```python
from build123d import *

# Parameters (mm, degrees)
BOSS_EXTRUDE1_DEPTH = 17
SKETCH3_R           = 3.25
CUT_EXTRUDE1_DEPTH  = 6
SKETCH4_R           = 3
BOSS_EXTRUDE2_DEPTH = 8


with BuildPart() as part:
    # Sketch2 → Boss-Extrude1 (new body)
    with BuildSketch(Plane.XY):
        with BuildLine():
            Line((-50.590688259, -20.348178138), (79.409311741, -20.348178138))
            ThreePointArc((79.409311741, -20.348178138), (86.480379553, -17.41924595), (89.409311741, -10.348178138))
            Line((89.409311741, -10.348178138), (89.409311741, -5.348178138))
            Line((89.409311741, -5.348178138), (79.409311741, -5.348178138))
            Line((79.409311741, -5.348178138), (69.749311741, -5.348178138))
            Line((69.749311741, -5.348178138), (69.749311741, -15.348178138))
            Line((69.749311741, -15.348178138), (34.109311741, -15.348178138))
            Line((34.109311741, -15.348178138), (34.109311741, -5.348178138))
            Line((34.109311741, -5.348178138), (-50.590688259, -5.348178138))
            Line((-50.590688259, -5.348178138), (-60.590688259, -5.348178138))
            Line((-60.590688259, -5.348178138), (-60.590688259, -10.348178138))
            ThreePointArc((-60.590688259, -10.348178138), (-57.661756071, -17.41924595), (-50.590688259, -20.348178138))
        make_face()
    extrude(amount=BOSS_EXTRUDE1_DEPTH)

    # Sketch3 → Cut-Extrude1 (cut)
    with BuildSketch(Plane(origin=(0, 0, 0), x_dir=(-1, 0, 0), z_dir=(0, 0, -1))):
        with Locations((-14.409311741, -12.848178138)):
            Circle(SKETCH3_R)
        with Locations((51.590688259, -12.848178138)):
            Circle(SKETCH3_R)
    extrude(amount=-CUT_EXTRUDE1_DEPTH, mode=Mode.SUBTRACT)

    # Sketch4 → Boss-Extrude2 (add)
    with BuildSketch(Plane.XY.offset(17)):
        with Locations((-51.590688259, -12.848178138)):
            Circle(SKETCH4_R)
    extrude(amount=BOSS_EXTRUDE2_DEPTH)


solid = part.part
```
Can you work these out from the model? Positions are in its coordinate system, mm. A direction names the side the tool comes from. Give positions to 0.01 mm unless a question says otherwise; leave off trailing zeros. Loops run counter-clockwise (first coordinate to the right, second up) from the corner with the lowest first, then second, coordinate; pieces in that order, holes last. Notation, with made-up numbers: M 79,77 L 132,77 A20 ccw 132,91 Z; hole C 29.5,29 d3. An arc over 180 degrees is marked long. Use CSV: the item, a comma, the result in double quotes. Start each with the question number.
1. On a 3-axis mill with a long thin cutter (end or side, diameter ignored), from which of +Z, -Z, +X, -X, +Y, -Y can I reach the whole of each face in a straight line? I mean faces 1 (the face through (86.4, -17.5, 8.4)), 2 (the face through (-57.74, -17.34, 8.38)), 3 (the face through (-48.73, -11.95, 20.94)), 4 (the face through (-54.593, -14.093, 2.958)), 5 (the face through (34.109, -10, 8)). Say none if no direction works.
2. Imagine slicing it at B-B, the plane z = 7.75. Write out the boundary of the cut face in (x, y), plus the area to 3 significant figures.
3. Imagine slicing it at A-A, the plane y = -8. Write out the boundary of the cut face in (x, z), plus the area to 3 significant figures.
4. Imagine slicing it at C-C, the plane x = -28.5. Write out the boundary of the cut face in (y, z), plus the area to 3 significant figures.
5. If we mould it in two halves opening along Y, with no side actions, what happens to faces 6 (the face through (13, -16, 0)), 7 (the face through (14, -13, 6)), 8 (the face through (80, -5.348, 8)), 9 (the face through (-52, -13, 6))? For each: released by +Y, released by -Y, zero draft, split by the parting line, or undercut.
6. Imagine slicing it at D-D, the plane y = -18. Write out the boundary of the cut face in (x, z).
7. If I drill on L1, parallel to X at y = -15.75, z = 4; L2, parallel to X at y = -10, z = 4; L3, parallel to X at y = -8, z = 7, over which ranges is the centre line in solid material (lowest first)?
8. For P1, Ø7.5, axis at x = 14.41, y = -12.85, coming from the +Z side; P2, Ø2, axis at x = 15.5, y = -11.5, coming from the -Z side; P3, Ø5, axis at x = 46.5, y = -12.5, coming from the +Z side, each with a flat end and sliding along its axis, tell me the tip position at first contact or that it passes through.
Response values:
1,face 1,"+Z, -Z, +X, -Y"
1,face 2,"+Z, -Z, -X, -Y"
1,face 3,"+Z"
1,face 4,"-Z"
1,face 5,"+Z, -Z, +Y"
2,outline,"M -60.59,-10.35 A10 ccw -50.59,-20.35 L 79.41,-20.35 A10 ccw 89.41,-10.35 L 89.41,-5.35 L 69.75,-5.35 L 69.75,-15.35 L 34.11,-15.35 L 34.11,-5.35 L -60.59,-5.35 Z"
2,area,"1,850 mm^2"
3,outline,"M -60.59,0 L 34.11,0 L 34.11,17 L -60.59,17 Z; M 69.75,0 L 89.41,0 L 89.41,17 L 69.75,17 Z"
3,area,"1,940 mm^2"
4,outline,"M -20.35,0 L -5.35,0 L -5.35,17 L -20.35,17 Z"
4,area,"255 mm^2"
5,face 6,"zero draft"
5,face 7,"undercut"
5,face 8,"released by +Y"
5,face 9,"undercut"
6,outline,"M -57.03,0 L 85.85,0 L 85.85,17 L -57.03,17 Z"
7,L1,"-59.01 to -53.05, -50.13 to 12.95, 15.87 to 87.82"
7,L2,"-60.59 to -53.16, -50.03 to 12.84, 15.97 to 34.11, 69.75 to 89.41"
7,L3,"-60.59 to 34.11, 69.75 to 89.41"
8,P1,"z = 17"
8,P2,"z = 6"
8,P3,"through"
